from build123d import *

# Parameters (mm, degrees)
BOSS_EXTRUDE1_DEPTH = 135.3879
SKETCH2_R           = 2.155
SKETCH2_W           = 30
SKETCH2_H           = 20
CUT_EXTRUDE1_DEPTH  = 1.6002


with BuildPart() as part:
    # Sketch1 → Boss-Extrude1 (new body)
    with BuildSketch(Plane(origin=(0, 0, 0), x_dir=(0, 0, -1), z_dir=(1, 0, 0))):
        Polygon((0, 0), (0, -1.6002), (50, -1.6002), (50, -89.49088), (0, -89.49088), (0, -91.09108), (51.6002, -91.09108), (51.6002, 0), align=None)
    extrude(amount=BOSS_EXTRUDE1_DEPTH)

    # Sketch2 → Cut-Extrude1 (cut)
    with BuildSketch(Plane.XY.offset(-50)):
        with Locations((42.69395, -25.54554)):
            Circle(SKETCH2_R)
        with Locations((92.69395, -25.54554)):
            Circle(SKETCH2_R)
        with Locations((42.69395, -45.54554)):
            Circle(SKETCH2_R)
        with Locations((92.69395, -45.54554)):
            Circle(SKETCH2_R)
        with Locations((67.69395, -43.54554)):
            Rectangle(SKETCH2_W, SKETCH2_H)
    extrude(amount=-CUT_EXTRUDE1_DEPTH, mode=Mode.SUBTRACT)


solid = part.part
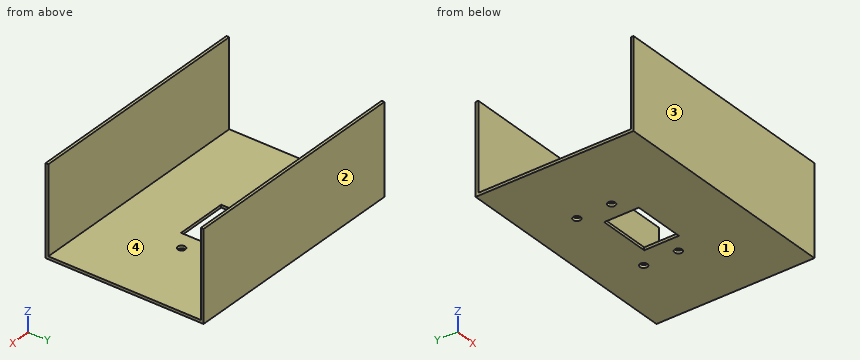
Can you work these out from the model? Positions are in its coordinate system, mm. Face numbers are marked on the shaded views. Coordinates: 2 decimals unless noted, no trailing zeros. Write each loop counter-clockwise with the first axis right and the second up, starting at its lowest first coordinate (ties: lowest second). Pieces come first, ordered by that corner, then holes. Notation, with made-up numbers: (54, 21) -> (66, 21) arc R34 ccw to (66, 54) -> close; hole circle Ø5 at (72.25, -38). An arc over 180 degrees is marked (long way). Answer as CSV lines item,"result".
1) Will these pins go through, and if not, where does the flat tip stop? P1, Ø8, axis at x = 56.5, y = -51, coming from the +Z side; P2, Ø0.5, axis at x = 69, z = -50.5, coming from the +Y side; P3, Ø4, axis at x = 92.69, y = -45.55, coming from the -Z side.
Check result:
P1,"z = -50"
P2,"y = 0"
P3,"through"
2) If I drill on line 1 (Y direction, x = 39, z = -19); line 2 (Z direction, x = 9, y = -45), over which ranges is the centre line in solid material (lowest first)? Write a range as from..to.
Check result:
line 1,"-91.09..-89.49, -1.6..0"
line 2,"-51.6..-50"
3) If we section it at C-C on y = -51: Please give me the cut outline in (x, z).
Check result:
outline,"(0, -51.6) -> (52.69, -51.6) -> (52.69, -50) -> (0, -50) -> close; (82.69, -51.6) -> (135.39, -51.6) -> (135.39, -50) -> (82.69, -50) -> close"
4) If we section it at B-B on z = -35: Please give me the cut outline in (x, y), then the cut area to 3 significant figures.
Check result:
outline,"(0, -91.09) -> (135.39, -91.09) -> (135.39, -89.49) -> (0, -89.49) -> close; (0, -1.6) -> (135.39, -1.6) -> (135.39, 0) -> (0, 0) -> close"
area,"433 mm²"
5) If we mould it in two halves opening along Y, with no side actions, what happens to the marked faces 1, 2, 3 and 4? For each: +Y half, -Y half, draft (parallel to the pull), parting line (faces both ways), or undercut.
Check result:
face 1,"draft"
face 2,"+Y half"
face 3,"-Y half"
face 4,"undercut"
6) If we section it at A-A on x = 58.5: Please give me the cut outline in (y, z), then the cut area to 3 significant figures.
Check result:
outline,"(-91.09, -51.6) -> (-53.55, -51.6) -> (-53.55, -50) -> (-89.49, -50) -> (-89.49, 0) -> (-91.09, 0) -> close; (-33.55, -51.6) -> (0, -51.6) -> (0, 0) -> (-1.6, 0) -> (-1.6, -50) -> (-33.55, -50) -> close"
area,"274 mm²"
7) If we section it at D-D on x = 110.5: Please give me the cut outline in (y, z).
Check result:
outline,"(-91.09, -51.6) -> (0, -51.6) -> (0, 0) -> (-1.6, 0) -> (-1.6, -50) -> (-89.49, -50) -> (-89.49, 0) -> (-91.09, 0) -> close"
